Input: part model. Units: mm. Frame: model coordinates. A direction names the side the tool comes from. Round coordinates to 2 decimals unless told otherwise and drop trailing zeros. Write each loop counter-clockwise with the first axis right and the second up, starting at its lowest first coordinate (ties: lowest second). Pieces come first, ordered by that corner, then holes. Notation, with made-up numbers: (52.25, 89.5) -> (99.25, 89.5) arc R25 cw to (99.25, 120.5) -> close; hole circle Ø7 at (49, 36.5). An arc over 180 degrees is marked (long way). Write item = value, one per line. Start each with the question number.
Autodesk Inventor part; units mm, degrees
ref_plane "YZ Plane" through (0, 0, 0) normal (1, 0, 0) x (0, 1, 0)
ref_plane "XZ Plane" through (0, 0, 0) normal (0, 1, 0) x (-1, 0, 0)
ref_plane "XY Plane" through (0, 0, 0) normal (0, 0, 1) x (1, 0, 0)
sketch "Sketch1" plane through (0, 0, 0) normal (0, 0, 1) x (1, 0, 0)
  line L0 (0, 3.5) -> (0, -3.5)
  line L1 (0, -3.5) -> (1.25, -3.5)
  line L2 (1.25, -3.5) -> (1.5, -3.25)
  line L3 (1.5, -3.25) -> (1.5, 2.4)
  line L4 (1.6, 2.5) -> (2.75, 2.5)
  line L5 (2.75, 2.5) -> (2.75, 3.35)
  line L6 (2.6, 3.5) -> (0, 3.5)
  arc A0 (1.6, 2.5) -> (1.5, 2.4) centre (1.6, 2.4) ccw
  line L7 (2.6, 3.5) -> (2.75, 3.35)
  point P0 (0, 0)
  point P1 (2.75, 3.5)
  point P2 (0, 0)
  dimension "d0" = 5.5
  dimension "d1" = 1
  dimension "d3" = 3
  dimension "d4" = 3.2
  dimension "d5" = 135
  dimension "d6" = 0.25
  dimension "d7" = 6
  dimension "d18" = 0.15
  dimension "d22" = 0.15
revolve "Revolution1" add sketch "Sketch1" angle 360 about axis through (0, 3.5, 0) along (0, -1, 0)
sketch "Sketch2" plane through (0, 3.5, 0) normal (0, 1, 0) x (1, 0, 0)
  line L0 (0, -1.1547) -> (-1, -0.5774)
  line L1 (-1, -0.5774) -> (-1, 0.5774)
  line L2 (-1, 0.5774) -> (0, 1.1547)
  line L3 (0, 1.1547) -> (1, 0.5774)
  line L4 (1, 0.5774) -> (1, -0.5774)
  line L5 (1, -0.5774) -> (0, -1.1547)
  point P0 (0, 0)
  point P1 (0, 0)
  dimension "d11" = 2
extrude "Extrusion1" cut sketch "Sketch2" against normal blind 1
thread "Thread1"
sketch "Sketch3" plane through (0, 0, 0) normal (1, 0, 0) x (0, 1, 0)
  line L0 (3.5, 1.1547) -> (3.5, 0.5774)
  line L1 (3.5, 1.1547) -> (3, 0.6547)
  line L2 (3, 0.6547) -> (3.5, 0.6547)
  line L3 (3.5, 0.6547) -> (3.5, 1.1547)
  line L4 (-0.9, 0) -> (5.4, 0)
  point P0 (0, 0)
  dimension "d16" = 0.5
revolve "Revolution2" cut sketch "Sketch3" angle 360 about axis through (0, -10, 0) along (0, 1, 0)
equation "\"d22\" = d18"
properties part number "48-0362" material "Stainless Steel"
1. Section B-B (z = 0). Output: boundary loops of the cut face in (x, y), then the cut area to 3 significant figures.
2. Reachability of faces 1 (the flat face through (0.51, 3.01, 0.86)), 2 (the flat face through (0, -3.5, 0)), 3 (the flat face through (2, 2.5, 0)) from +Z, -Z, +X, -X, +Y, -Y: full face, straight path, thin tool, end or side. Return the list, or none.
3. Section C-C (y = 1). Output: boundary loops of the cut face in (x, z), then the cut area to 3 significant figures.
4. Mould query, pull axis Z, two halves, no side actions, for faces 4 (the flat face through (1, 3.5, -1)), 5 (the flat face through (-1, 3, 0)), 6 (the cylindrical face through (-0.596, 2.931, 2.685)). Classes: pulls with the +Z half, pulls with the -Z half, needs draft (parallel to the pull), parting line crosses it, or undercut.
5. Section A-A (y = 2.75). Output: boundary loops of the cut face in (x, z), then the cut area to 3 significant figures.
6. Line query: line 1 along Y through (x, z) = (0.4, 2.4); line 2 along Y through (x, z) = (-0.7, 0.5); line 3 along Z through (x, y) = (0, -3). Output: solid intervals per line, ascending.
7. Pin query (flat end, axial travel): P1, Ø0.6, axis at x = 0, z = -0.5, coming from the +Y side; P2, Ø1.5, axis at x = 1, y = 2.5, coming from the +Z side. Return the tip coordinate at first contact, or that it passes through.
Check sheet entries:
q1.outline = (-2.75, 2.5) -> (-1.6, 2.5) arc R0.1 cw to (-1.5, 2.4) -> (-1.5, -3.25) -> (-1.25, -3.5) -> (1.25, -3.5) -> (1.5, -3.25) -> (1.5, 2.4) arc R0.1 cw to (1.6, 2.5) -> (2.75, 2.5) -> (2.75, 3.35) -> (2.6, 3.5) -> (1.15, 3.5) -> (1, 3.35) -> (1, 2.5) -> (-1, 2.5) -> (-1, 3.35) -> (-1.15, 3.5) -> (-2.6, 3.5) -> (-2.75, 3.35) -> close
q1.area = 21.4 mm2
q2.face_1 = +Y
q2.face_2 = +Z, -Z, +X, -X, -Y
q2.face_3 = -Y
q3.outline = circle Ø3 at (0, 0)
q3.area = 7.07 mm2
q4.face_4 = needs draft
q4.face_5 = undercut
q4.face_6 = parting line crosses it
q5.outline = circle Ø5.5 at (0, 0); hole (-1, -0.58) -> (0, -1.15) -> (1, -0.58) -> (1, 0.58) -> (0, 1.15) -> (-1, 0.58) -> close
q5.area = 20.3 mm2
q6.line_1 = 2.5 to 3.5
q6.line_2 = -3.5 to 2.5
q6.line_3 = -1.5 to 1.5
q7.P1 = 2.5
q7.P2 = 2.74
